from build123d import *

# Parameters (mm, degrees)
SKETCH_W        = 40
SKETCH_H        = 40
PAD_DEPTH       = 20
SKETCH001_R     = 6
POCKET_DEPTH    = 33
SKETCH002_R     = 3.1
POCKET001_DEPTH = 8
SKETCH003_R     = 6
POCKET002_DEPTH = 33
SKETCH004_R     = 3.1
POCKET003_DEPTH = 8
POCKET004_DEPTH = 25
FILLET_R        = 2
FILLET001_R     = 2
FILLET002_R     = 2
FILLET003_R     = 1
FILLET004_R     = 1


with BuildPart() as part:
    # Sketch → Pad (new body)
    with BuildSketch(Plane.XY):
        with Locations((20, 20)):
            Rectangle(SKETCH_W, SKETCH_H)
    extrude(amount=PAD_DEPTH)

    # Sketch001 → Pocket (cut)
    with BuildSketch(Plane.XZ):
        with Locations((20, 10)):
            Circle(SKETCH001_R)
    extrude(amount=-POCKET_DEPTH, mode=Mode.SUBTRACT)

    # Sketch002 → Pocket001 (cut)
    with BuildSketch(Plane.XZ.offset(-33)):
        with Locations((20, 10)):
            Circle(SKETCH002_R)
    extrude(amount=-POCKET001_DEPTH, mode=Mode.SUBTRACT)

    # Sketch003 → Pocket002 (cut)
    with BuildSketch(Plane.YZ.offset(40)):
        with Locations((20, 10)):
            Circle(SKETCH003_R)
    extrude(amount=-POCKET002_DEPTH, mode=Mode.SUBTRACT)

    # Sketch004 → Pocket003 (cut)
    with BuildSketch(Plane.YZ.offset(7)):
        with Locations((20, 10)):
            Circle(SKETCH004_R)
    extrude(amount=-POCKET003_DEPTH, mode=Mode.SUBTRACT)

    # Sketch005 → Pocket004 (cut)
    with BuildSketch(Plane.XY.offset(20)):
        Polygon((0, 0), (40, 40), (40, 0), align=None)
    extrude(amount=-POCKET004_DEPTH, mode=Mode.SUBTRACT)

    # Fillet
    fillet_edges = [part.edges().sort_by_distance(p)[0] for p in [
        (40, 40, 10),
    ]]
    fillet(fillet_edges, radius=FILLET_R)

    # Fillet001
    fillet001_edges = [part.edges().sort_by_distance(p)[0] for p in [
        (0, 0, 10),
    ]]
    fillet(fillet001_edges, radius=FILLET001_R)

    # Fillet002
    fillet002_edges = [part.edges().sort_by_distance(p)[0] for p in [
        (0, 40, 10),
    ]]
    fillet(fillet002_edges, radius=FILLET002_R)

    # Fillet003
    fillet003_edges = [part.edges().sort_by_distance(p)[0] for p in [
        (0, 21.414214, 0),
        (0.585786, 39.414214, 0),
        (1.234633, 2.980668, 0),
        (18.585786, 40, 0),
        (20, 20, 0),
        (37.019332, 38.765367, 0),
    ]]
    fillet(fillet003_edges, radius=FILLET003_R)

    # Fillet004
    fillet004_edges = [part.edges().sort_by_distance(p)[0] for p in [
        (0, 21.414214, 20),
        (0.585786, 39.414214, 20),
        (1.234633, 2.980668, 20),
        (18.585786, 40, 20),
        (20, 20, 20),
        (37.019332, 38.765367, 20),
    ]]
    fillet(fillet004_edges, radius=FILLET004_R)


solid = part.part
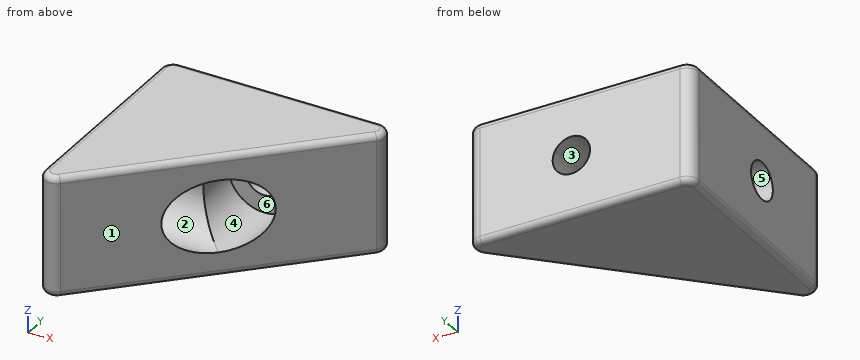
Part model, mm, in its own coordinate system. Face numbers are marked on the shaded views. A direction names the side the tool comes from. Coordinates: 2 decimals unless noted, no trailing zeros. Loops run counter-clockwise (first coordinate to the right, second up) from the corner with the lowest first, then second, coordinate; pieces in that order, holes last. Notation, with made-up numbers: (5, -29.75) -> (46, -29.75) arc R30 ccw to (46, -7.75) -> close; hole circle Ø4 at (-1.5, -26). An arc over 180 degrees is marked (long way). Use a Markdown table: item, result. Add a question column.
Item 1: Flat gauge pins, fed straight in: P1, Ø6, axis at y = 19, z = 9, coming from the +X side; P2, Ø5, axis at x = 6.5, z = 5, coming from the -Y side; P3, Ø6, axis at x = 21.5, z = 15, coming from the -Y side. Where does each tip first touch, or does it go through?
Item 2: Which spindle directions (+Z, -Z, +X, -X, +Y, -Y) get a long thin tool onto all of the face, cutting with end or side? Do the marked faces 5 and 6. Say none if no direction does.
Item 3: Band-saw the part on B-B on z = 17.5. Write the cut outline in (x, y).
Item 4: Probe probe 1 along Z at (x, y) = (10, 20); probe 2 along Z at (x, y) = (3, 20); probe 3 along Y at (x, z) = (25.5, 9.25). List the from-to ranges inside material, lowest first.
Item 5: Pull direction X, two halves, no side cores. Call the marked faces 1, 2, 3 and 4: +X half, -X half, draft (parallel to the pull), parting line (faces both ways), or undercut.
Item 6: Band-saw the part on C-C on z = 6.25. Write the cut outline in (x, y).
Item 7: Band-saw the part on A-A on z = 10. Write the cut outline in (x, y), plus the area to 3 significant figures.
Geometry says:
| question | item | result |
|---|---|---|
| 1 | P1 | x = 7 |
| 1 | P2 | y = 4 |
| 1 | P3 | y = 18.62 |
| 2 | face 5 | +X, -X |
| 2 | face 6 | -Y |
| 3 | outline | (0, 4.83) arc R2 ccw to (3.41, 3.41) -> (36.59, 36.59) arc R2 ccw to (35.17, 40) -> (2, 40) arc R2 ccw to (0, 38) -> close |
| 4 | probe 1 | 0 to 4, 16 to 20 |
| 4 | probe 2 | 0 to 6.9, 13.1 to 20 |
| 4 | probe 3 | 33 to 40 |
| 5 | face 1 | +X half |
| 5 | face 2 | draft |
| 5 | face 3 | undercut |
| 5 | face 4 | undercut |
| 6 | outline | (0, 4.83) arc R2 ccw to (3.41, 3.41) -> (15.32, 15.32) -> (7, 15.32) -> (7, 24.68) -> (15.32, 24.68) -> (15.32, 33) -> (24.68, 33) -> (24.68, 24.68) -> (36.59, 36.59) arc R2 ccw to (35.17, 40) -> (2, 40) arc R2 ccw to (0, 38) -> close |
| 7 | outline | (0, 4.83) arc R2 ccw to (3.41, 3.41) -> (14, 14) -> (7, 14) -> (7, 16.9) -> (0, 16.9) -> close; (0, 23.1) -> (7, 23.1) -> (7, 26) -> (14, 26) -> (14, 33) -> (16.9, 33) -> (16.9, 40) -> (2, 40) arc R2 ccw to (0, 38) -> close; (23.1, 33) -> (26, 33) -> (26, 26) -> (36.59, 36.59) arc R2 ccw to (35.17, 40) -> (23.1, 40) -> close |
| 7 | area | 462 mm² |
